from build123d import *

# Parameters (mm, degrees)
SKETCH_1_W          = 74
SKETCH_1_H          = 24
EXTRUDE_1_DEPTH     = 380
SKETCH_2_W          = 51.146480438
SKETCH_2_H          = 42.897874587
CUT_EXTRUDE_1_DEPTH = 381
SKETCH_3_OUTSIDE_W  = 108.472
SKETCH_3_OUTSIDE_H  = 458.472
CUT_EXTRUDE_2_DEPTH = 31


with BuildPart() as part:
    # Эскиз1 → Вытянуть-Тонкостенный1 (new body)
    with BuildSketch(Plane(origin=(0, 0, 0), x_dir=(1, 0, 0), z_dir=(0, 1, 0))):
        with BuildLine():
            Line((40, 12), (40, -12))
            ThreePointArc((40, -12), (39.121320344, -14.121320344), (37, -15))
            Line((37, -15), (-37, -15))
            ThreePointArc((-37, -15), (-39.121320344, -14.121320344), (-40, -12))
            Line((-40, -12), (-40, 12))
            ThreePointArc((-40, 12), (-39.121320344, 14.121320344), (-37, 15))
            Line((-37, 15), (37, 15))
            ThreePointArc((37, 15), (39.121320344, 14.121320344), (40, 12))
        make_face()
        Rectangle(SKETCH_1_W, SKETCH_1_H, mode=Mode.SUBTRACT)
    extrude(amount=EXTRUDE_1_DEPTH)

    # Эскиз2 → Вырез-Вытянуть1 (cut, through all)
    with BuildSketch(Plane(origin=(0, 380, 0), x_dir=(1, 0, 0), z_dir=(0, 1, 0))):
        with Locations((15.573240219, -0.476163575)):
            Rectangle(SKETCH_2_W, SKETCH_2_H)
    extrude(amount=-CUT_EXTRUDE_1_DEPTH, mode=Mode.SUBTRACT)

    # Эскиз3 outside → Вырез-Вытянуть2 (cut, through all)
    with BuildSketch(Plane.XY.offset(15)):
        with Locations((-25, 190)):
            Rectangle(SKETCH_3_OUTSIDE_W, SKETCH_3_OUTSIDE_H)
        Polygon((-40, 380), (-10, 188.075345928), (-10, 4.689340222), (-40, 0), align=None, mode=Mode.SUBTRACT)
    extrude(amount=-CUT_EXTRUDE_2_DEPTH, mode=Mode.SUBTRACT)


solid = part.part
Source: CAD feature listing. Evaluate the final solid. Frame: model axes, mm. A direction names the side the tool comes from. Give positions to 0.01 mm unless a question says otherwise; leave off trailing zeros. Loops run counter-clockwise (first coordinate to the right, second up) from the corner with the lowest first, then second, coordinate; pieces in that order, holes last. Notation, with made-up numbers: (-28.5, 50.5) -> (-23.5, 50.5) arc R17 cw to (-23.5, 83.5) -> close; hole circle Ø4 at (57.25, -26). An arc over 180 degrees is marked (long way). Use a Markdown table: item, result. Add a question column.
1) Reachability of faces 4 (the face through (-24, 138, 12)), 5 (the face through (-28.4, 305.8, 12.3)) from +Z, -Z, +X, -X, +Y, -Y: full face, straight path, thin tool, end or side. Return the list, or none.
2) Section query B-B, the plane y = 81. Return the cut outline in (x, z), then the cut area to 3 significant figures.
3) Pull-direction query (Z, two-part tool) for faces 1 (the face through (-24, 138, -12)), 2 (the face through (-37.152, 0.445, 0.07)), 3 (the face through (-23, 138, 15)); classes: +Z half, -Z half, draft (parallel to the pull), parting line (faces both ways), or undercut.
4) Section query C-C, the plane x = -31.5. Return the cut outline in (y, z), then the cut area to 3 significant figures.
5) First-contact query: pin 1 (10 mm diameter, centred on y = 146.5, z = 8.5, fed in from +X); pin 2 (4 mm diameter, centred on y = 160, z = 2.5, fed in from +X). Flat tips, straight axial feed; report the tip coordinate or a pass-through.
6) Line query: line 1 along Z through (x, y) = (-11.5, 114); line 2 along X through (y, z) = (360.5, -2); line 3 along X through (y, z) = (195.5, 14). Output: solid intervals per line, ascending. Write a range as [from, to].
7) Section query D-D, the plane z = 0. Return the cut outline in (x, y), then the cut area to 3 significant figures.
8) Section query A-A, the plane x = -17.5. Return the cut outline in (y, z), then the cut area to 3 significant figures.
Numbers:
| question | item | result |
|---|---|---|
| 1 | face 4 | +X, +Y, -Y |
| 1 | face 5 | +Z, -Z, +X, +Y |
| 2 | outline | (-40, -12) arc R3 ccw to (-37, -15) -> (-10, -15) -> (-10, -12) -> (-37, -12) -> (-37, 12) -> (-10, 12) -> (-10, 15) -> (-37, 15) arc R3 ccw to (-40, 12) -> close |
| 2 | area | 248 mm2 |
| 3 | face 1 | undercut |
| 3 | face 2 | draft |
| 3 | face 3 | +Z half |
| 4 | outline | (1.33, -15) -> (325.62, -15) -> (325.62, -12) -> (1.33, -12) -> close; (1.33, 12) -> (325.62, 12) -> (325.62, 15) -> (1.33, 15) -> close |
| 4 | area | 1,950 mm2 |
| 5 | pin 1 | stops at x = -10 |
| 5 | pin 2 | stops at x = -37 |
| 6 | line 1 | z = [-15, -12], [12, 15] |
| 6 | line 2 | x = [-40, -37] |
| 6 | line 3 | x = [-39.24, -11.16] |
| 7 | outline | (-40, 0) -> (-37, 0.47) -> (-37, 360.81) -> (-40, 380) -> close |
| 7 | area | 1,110 mm2 |
| 8 | outline | (3.52, -15) -> (236.06, -15) -> (236.06, -12) -> (3.52, -12) -> close; (3.52, 12) -> (236.06, 12) -> (236.06, 15) -> (3.52, 15) -> close |
| 8 | area | 1,400 mm2 |
